Could you check a few things on this model? Use its own coordinates, in mm. Face numbers are marked on the shaded views. A direction names the side the tool comes from. Round coordinates to 2 decimals unless told otherwise and drop trailing zeros. Order: outer loops, then holes, each group sorted by start corner. A loop starts at its lowest first (then second) coordinate and runs counter-clockwise, first axis right, second up. Notation, with made-up numbers: (65.25, 59) -> (102.25, 59) arc R16 ccw to (102.25, 69) -> close; hole circle Ø5 at (-11.5, 53). An arc over 180 degrees is marked (long way). One line per question, with ' | ' between items.
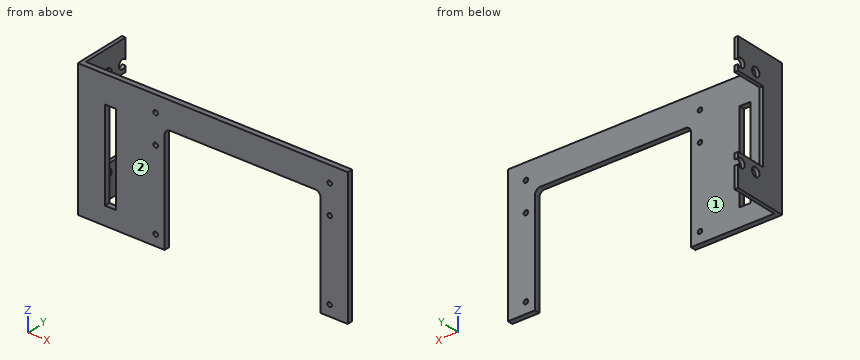
```python
from build123d import *

# Parameters (mm, degrees)
SKETCH_1_R          = 1.25
EXTRUDE_1_DEPTH     = 3
FILLET_1_R          = 3
SKETCH_2_W          = 75
SKETCH_2_H          = 3
EXTRUDE_2_DEPTH     = 32.9
SKETCH_3_W          = 2
SKETCH_3_H          = 75
EXTRUDE_4_DEPTH     = 30
CUT_EXTRUDE_1_REACH = 164.076
SKETCH_5_W          = 40.1
SKETCH_5_H          = 20.1
CUT_EXTRUDE_2_REACH = 165.891
SKETCH_6_R          = 2.5
SKETCH_7_W          = 2
SKETCH_7_H          = 75
CUT_EXTRUDE_3_DEPTH = 3
SKETCH_9_W          = 6
SKETCH_9_H          = 50
CUT_EXTRUDE_4_DEPTH = 121.540449642


with BuildPart() as part:
    # 草图1 → 凸台-拉伸1 (new body)
    with BuildSketch(Plane(origin=(0, 0, 0), x_dir=(1, 0, 0), z_dir=(0, 1, 0))):
        Polygon((0, 0), (0, 60), (-15, 60), (-15, -15), (101, -15), (101, 60), (86, 60), (86, 0), align=None)
        with Locations(Location((-5, 54, 0), (0, 0, 270))):
            Circle(SKETCH_1_R, mode=Mode.SUBTRACT)
        with Locations(Location((-5, -6, 0), (0, 0, 90))):
            Circle(SKETCH_1_R, mode=Mode.SUBTRACT)
        with Locations(Location((91, 54, 0), (0, 0, 270))):
            Circle(SKETCH_1_R, mode=Mode.SUBTRACT)
        with Locations(Location((91, -6, 0), (0, 0, 270))):
            Circle(SKETCH_1_R, mode=Mode.SUBTRACT)
        with Locations(Location((91, 10, 0), (0, 0, 270))):
            Circle(SKETCH_1_R, mode=Mode.SUBTRACT)
        with Locations(Location((-5, 10, 0), (0, 0, 90))):
            Circle(SKETCH_1_R, mode=Mode.SUBTRACT)
    extrude(amount=EXTRUDE_1_DEPTH)

    # 圆角1
    fillet_1_edges = [part.edges().sort_by_distance(p)[0] for p in [
        (86, 1.5, 0),
        (0, 1.5, 0),
    ]]
    fillet(fillet_1_edges, radius=FILLET_1_R)

    # 草图2 → 凸台-拉伸2 (add)
    with BuildSketch(Plane.ZY.offset(15)):
        with Locations((-22.5, 1.5)):
            Rectangle(SKETCH_2_W, SKETCH_2_H)
    extrude(amount=EXTRUDE_2_DEPTH)

    # 草图3 → 凸台-拉伸4 (add)
    with BuildSketch(Plane(origin=(0, 3, 0), x_dir=(1, 0, 0), z_dir=(0, 1, 0))):
        with Locations((-46.9, 22.5)):
            Rectangle(SKETCH_3_W, SKETCH_3_H)
    extrude(amount=EXTRUDE_4_DEPTH)

    # 草图5 → 切除-拉伸1 (cut, up to next)
    with BuildSketch(Plane(origin=(-45.9, 0, 0), x_dir=(0, 0, -1), z_dir=(1, 0, 0)), mode=Mode.PRIVATE) as cut_extrude_1_sk1:
        with Locations((22.15, 22.95)):
            Rectangle(SKETCH_5_W, SKETCH_5_H)
    cut_extrude_1_tool1 = extrude(cut_extrude_1_sk1.sketch, amount=-CUT_EXTRUDE_1_REACH, mode=Mode.PRIVATE) & part.part
    add(cut_extrude_1_tool1.solids().sort_by_distance((-45.9, 22.95, -22.15))[0], mode=Mode.SUBTRACT)

    # 草图6 → 切除-拉伸2 (cut, up to next)
    with BuildSketch(Plane.ZY.offset(47.9), mode=Mode.PRIVATE) as cut_extrude_2_sk1:
        with Locations(Location((-46.85, 18, 0), (0, 0, 270))):
            Circle(SKETCH_6_R)
    cut_extrude_2_tool1 = extrude(cut_extrude_2_sk1.sketch, amount=-CUT_EXTRUDE_2_REACH, mode=Mode.PRIVATE) & part.part
    # 草图6 → 切除-拉伸2 (cut, up to next)
    with BuildSketch(Plane.ZY.offset(47.9), mode=Mode.PRIVATE) as cut_extrude_2_sk2:
        with Locations(Location((-46.85, 28, 0), (0, 0, 270))):
            Circle(SKETCH_6_R)
    cut_extrude_2_tool2 = extrude(cut_extrude_2_sk2.sketch, amount=-CUT_EXTRUDE_2_REACH, mode=Mode.PRIVATE) & part.part
    # 草图6 → 切除-拉伸2 (cut, up to next)
    with BuildSketch(Plane.ZY.offset(47.9), mode=Mode.PRIVATE) as cut_extrude_2_sk3:
        with Locations(Location((2.65, 18, 0), (0, 0, 270))):
            Circle(SKETCH_6_R)
    cut_extrude_2_tool3 = extrude(cut_extrude_2_sk3.sketch, amount=-CUT_EXTRUDE_2_REACH, mode=Mode.PRIVATE) & part.part
    # 草图6 → 切除-拉伸2 (cut, up to next)
    with BuildSketch(Plane.ZY.offset(47.9), mode=Mode.PRIVATE) as cut_extrude_2_sk4:
        with Locations(Location((2.65, 28, 0), (0, 0, 270))):
            Circle(SKETCH_6_R)
    cut_extrude_2_tool4 = extrude(cut_extrude_2_sk4.sketch, amount=-CUT_EXTRUDE_2_REACH, mode=Mode.PRIVATE) & part.part
    add(cut_extrude_2_tool1.solids().sort_by_distance((-47.9, 18, -46.85))[0], mode=Mode.SUBTRACT)
    add(cut_extrude_2_tool2.solids().sort_by_distance((-47.9, 28, -46.85))[0], mode=Mode.SUBTRACT)
    add(cut_extrude_2_tool3.solids().sort_by_distance((-47.9, 18, 2.65))[0], mode=Mode.SUBTRACT)
    add(cut_extrude_2_tool4.solids().sort_by_distance((-47.9, 28, 2.65))[0], mode=Mode.SUBTRACT)

    # 草图7 → 切除-拉伸3 (cut)
    with BuildSketch(Plane(origin=(0, 33, 0), x_dir=(1, 0, 0), z_dir=(0, 1, 0))):
        with Locations((-46.9, 22.5)):
            Rectangle(SKETCH_7_W, SKETCH_7_H)
    extrude(amount=-CUT_EXTRUDE_3_DEPTH, mode=Mode.SUBTRACT)

    # 草图9 → 切除-拉伸4 (cut, through all)
    with BuildSketch(Plane(origin=(0, 3, 0), x_dir=(1, 0, 0), z_dir=(0, 1, 0))):
        with Locations((-29.9, 25)):
            Rectangle(SKETCH_9_W, SKETCH_9_H)
    extrude(amount=-CUT_EXTRUDE_4_DEPTH, mode=Mode.SUBTRACT)


solid = part.part
```
1. I want a section at D-D on z = -46.85. List the corners of the cut face in (x, y) for me.
From the geometry:
outline: (-47.9, 0) -> (-32.9, 0) -> (-32.9, 3) -> (-45.9, 3) -> (-45.9, 15.5) -> (-47.9, 15.5) -> close; (-47.9, 20.5) -> (-45.9, 20.5) -> (-45.9, 25.5) -> (-47.9, 25.5) -> close; (-26.9, 0) -> (0, 0) -> (0, 3) -> (-26.9, 3) -> close; (86, 0) -> (101, 0) -> (101, 3) -> (86, 3) -> close
2. I need wall thicknesses on probe 1 along Z at (x, y) = (91, 1.95); probe 2 along X at (y, z) = (2, -54); probe 3 along X at (y, z) = (6.25, -21). Which ranges of each line are inside material? Lowest first, please.
From the geometry:
probe 1: z = -60 to -55.25, -52.75 to -11.25, -8.75 to 4.75, 7.25 to 15 | probe 2: x = -47.9 to -6.25, -3.75 to 0, 86 to 89.75, 92.25 to 101 | probe 3: x = -47.9 to -45.9
3. On a 3-axis mill with a long thin cutter (end or side, diameter ignored), from which of +Z, -Z, +X, -X, +Y, -Y can I reach the whole of each face in a straight line? I mean the marked faces 1 and 2. Say none if no direction works.
From the geometry:
face 1: +Z, -Z, +X, +Y | face 2: +Z, -Z, +X, -X, -Y
4. I want a section at B-B on y = 28. List the corners of the cut face in (x, z) for me, and give its area (3 significant figures).
From the geometry:
outline: (-47.9, -60) -> (-45.9, -60) -> (-45.9, -49.35) -> (-47.9, -49.35) -> close; (-47.9, -44.35) -> (-45.9, -44.35) -> (-45.9, -42.2) -> (-47.9, -42.2) -> close; (-47.9, -2.1) -> (-45.9, -2.1) -> (-45.9, 0.15) -> (-47.9, 0.15) -> close; (-47.9, 5.15) -> (-45.9, 5.15) -> (-45.9, 15) -> (-47.9, 15) -> close | area: 49.8 mm²
5. I want a section at C-C on z = -17. List the corners of the cut face in (x, y) for me, and give its area (4 significant figures).
From the geometry:
outline: (-47.9, 0) -> (-32.9, 0) -> (-32.9, 3) -> (-45.9, 3) -> (-45.9, 12.9) -> (-47.9, 12.9) -> close; (-26.9, 0) -> (0, 0) -> (0, 3) -> (-26.9, 3) -> close; (86, 0) -> (101, 0) -> (101, 3) -> (86, 3) -> close | area: 190.5 mm²
6. I want a section at A-A on z = 2.65. List the corners of the cut face in (x, y) for me, and give its area (3 significant figures).
From the geometry:
outline: (-47.9, 0) -> (101, 0) -> (101, 3) -> (-45.9, 3) -> (-45.9, 15.5) -> (-47.9, 15.5) -> close; (-47.9, 20.5) -> (-45.9, 20.5) -> (-45.9, 25.5) -> (-47.9, 25.5) -> close | area: 482 mm²
7. I'm going to push flat-ended pins straight in: pin 1 (8 mm diameter, centred on y = 20.5, z = -10, fed in from -X); pin 2 (6.5 mm diameter, centred on y = 18, z = 2.65, fed in from +X); pin 3 (10 mm diameter, centred on x = 35.5, y = 7, fed in from -Z); pin 4 (1.5 mm diameter, centred on x = -3.5, z = -40, fed in from +Y). Where does each tip first touch, or does it pass through?
From the geometry:
pin 1: passes through | pin 2: stops at x = -45.9 | pin 3: stops at z = 0 | pin 4: stops at y = 3
